from build123d import *

# Parameters (mm, degrees)
SKETCH1_W           = 30
SKETCH1_H           = 30
BOSS_EXTRUDE1_DEPTH = 350
SKETCH2_R           = 60
BOSS_EXTRUDE2_DEPTH = 80


with BuildPart() as part:
    # Sketch1 → Boss-Extrude1 (new body)
    with BuildSketch(Plane(origin=(0, 0, 0), x_dir=(1, 0, 0), z_dir=(0, 1, 0))):
        with Locations((0, 15)):
            Rectangle(SKETCH1_W, SKETCH1_H)
    extrude(amount=-BOSS_EXTRUDE1_DEPTH)

    # Sketch2 → Boss-Extrude2 (add)
    with BuildSketch(Plane.XZ.offset(350)):
        with Locations(Location((0, -15, 0), (0, 0, 270))):
            Circle(SKETCH2_R)
    extrude(amount=BOSS_EXTRUDE2_DEPTH)


solid = part.part
Model file for the job. Use its own axes, mm. A direction names the side the tool comes from. Give positions to 0.01 mm unless a question says otherwise; leave off trailing zeros. Order: outer loops, then holes, each group sorted by start corner. A loop starts at its lowest first (then second) coordinate and runs counter-clockwise, first axis right, second up. Notation, with made-up numbers: M 26,74.25 L 81,74.25 A22 cw 81,88.25 Z; hole C 20,-1 d1. An arc over 180 degrees is marked long. Write item = value, one per line.
Q1. Cut at A-A, the plane x = 0. List the corners of the cut face in (y, z), then the cut area to 3 significant figures.
Derived:
outline = M -430,-75 L -350,-75 L -350,-30 L 0,-30 L 0,0 L -350,0 L -350,45 L -430,45 Z
area = 20,100 mm2
Q2. Flat gauge pins, fed straight in: pin 1 (9 mm diameter, centred on y = -204, z = -22, fed in from +X); pin 2 (15 mm diameter, centred on x = -2, y = -99, fed in from +Z); pin 3 (9 mm diameter, centred on x = -3.5, y = -250, fed in from -Z). Where does each tip first touch, or does it go through?
Derived:
pin_1 = 15
pin_2 = 0
pin_3 = -30
Q3. Cut at B-B, the plane z = -15. List the corners of the cut face in (x, y).
Derived:
outline = M -60,-430 L 60,-430 L 60,-350 L 15,-350 L 15,0 L -15,0 L -15,-350 L -60,-350 Z
Q4. Drill centre lines: line 1 (Y direction, x = 18, z = 8); line 2 (X direction, y = -269.5, z = -26); line 3 (Z direction, x = 1.5, y = -204.5). Where is each one in solid material? Low to high. Write a range as [from, to].
Derived:
line_1 = [-430, -350]
line_2 = [-15, 15]
line_3 = [-30, 0]
Q5. Cut at D-D, the plane y = -32. List the corners of the cut face in (x, z).
Derived:
outline = M -15,-30 L 15,-30 L 15,0 L -15,0 Z
Q6. Cut at C-C, the plane y = -394. List the corners of the cut face in (x, z), then the cut area to 3 significant figures.
Derived:
outline = C 0,-15 d120
area = 11,300 mm2
Q7. Tool access for faces 1 (the flat face through (15, -173, -15)), 2 (the cylindrical face through (2.64, -389.44, 44.94)), 3 (the flat face through (0, -173, -30)), 4 (the flat face through (0, -173, 0)), 5 (the flat face through (-15, -173, -15)): list every direction of +Z, -Z, +X, -X, +Y, -Y with a clear straight run to the whole face (end or side of a thin tool).
Derived:
face_1 = +Z, -Z, +X, +Y
face_2 = +Y, -Y
face_3 = -Z, +X, -X, +Y
face_4 = +Z, +X, -X, +Y
face_5 = +Z, -Z, -X, +Y
